Geometry check sheet. Reference: drawing and pictorial views, mm from the part's lowest x, y, z. A direction names the side the tool comes from. Give positions to 0.01 mm unless a question says otherwise; leave off trailing zeros. Order: outer loops, then holes, each group sorted by start corner. A loop starts at its lowest first (then second) coordinate and runs counter-clockwise, first axis right, second up.
Item 1: Release check for a two-part mould opening along X. For the marked faces 3, 4 and 5 record: released by +X, released by -X, zero draft, split by the parting line, or undercut.
Item 2: Sectioned sample at A-A on x = 9. Record the boundary of the cut face in (y, z).
Item 3: Gauge pin test, flat ends, axial feed: P1, Ø1.5, axis at x = 5, z = 0.5, coming from the +Y side; P2, Ø1.5, axis at y = 14, z = 2.5, coming from the -X side. Record the tip position at first contact, or that the pin passes through.
Item 4: Material ranges on line 1 along Y through (x, z) = (9, 1.65); line 2 along Y through (x, z) = (9, 0.45); line 3 along Y through (x, z) = (9, 2.3), recorded low to high.
Item 5: Sectioned sample at C-C on x = 6.75. Record the boundary of the cut face in (y, z).
Item 6: Access from +Z, -Z, +X, -X, +Y, -Y to the whole of each face (thin tool, end or side, straight path). Record for the marked faces 1 and 2.
Item 7: Sectioned sample at D-D on y = 15. Record the boundary of the cut face in (x, z), and give its area (3 significant figures).
Item 8: Sectioned sample at B-B on y = 9. Record the boundary of the cut face in (x, z).
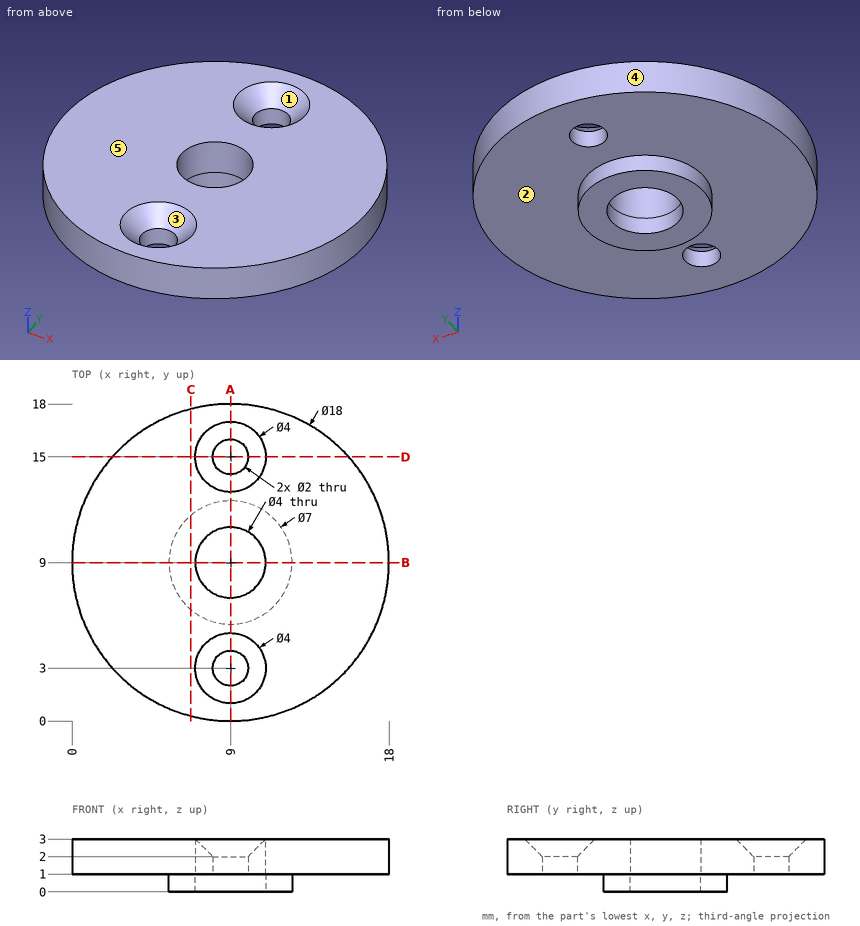
Report:
1. face 3: undercut
1. face 4: split by the parting line
1. face 5: zero draft
2. outline: (0, 1) - (2, 1) - (2, 2) - (1, 3) - (0, 3) - close; (4, 1) - (5.5, 1) - (5.5, 0) - (7, 0) - (7, 3) - (5, 3) - (4, 2) - close; (11, 0) - (12.5, 0) - (12.5, 1) - (14, 1) - (14, 2) - (13, 3) - (11, 3) - close; (16, 1) - (18, 1) - (18, 3) - (17, 3) - (16, 2) - close
3. P1: stops at y = 17.32
3. P2: stops at x = 1.07
4. line 1: y = 0 to 2, 4 to 7, 11 to 14, 16 to 18
4. line 2: y = 5.5 to 7, 11 to 12.5
4. line 3: y = 0 to 1.7, 4.3 to 7, 11 to 13.7, 16.3 to 18
5. outline: (0.29, 1) - (6.32, 1) - (6.32, 0) - (11.68, 0) - (11.68, 1) - (17.71, 1) - (17.71, 3) - (0.29, 3) - close
6. face 1: +Z
6. face 2: -Z
7. outline: (2.29, 1) - (8, 1) - (8, 2) - (7, 3) - (2.29, 3) - close; (10, 1) - (15.71, 1) - (15.71, 3) - (11, 3) - (10, 2) - close
7. area: 21.8 mm2
8. outline: (0, 1) - (5.5, 1) - (5.5, 0) - (7, 0) - (7, 3) - (0, 3) - close; (11, 0) - (12.5, 0) - (12.5, 1) - (18, 1) - (18, 3) - (11, 3) - close
